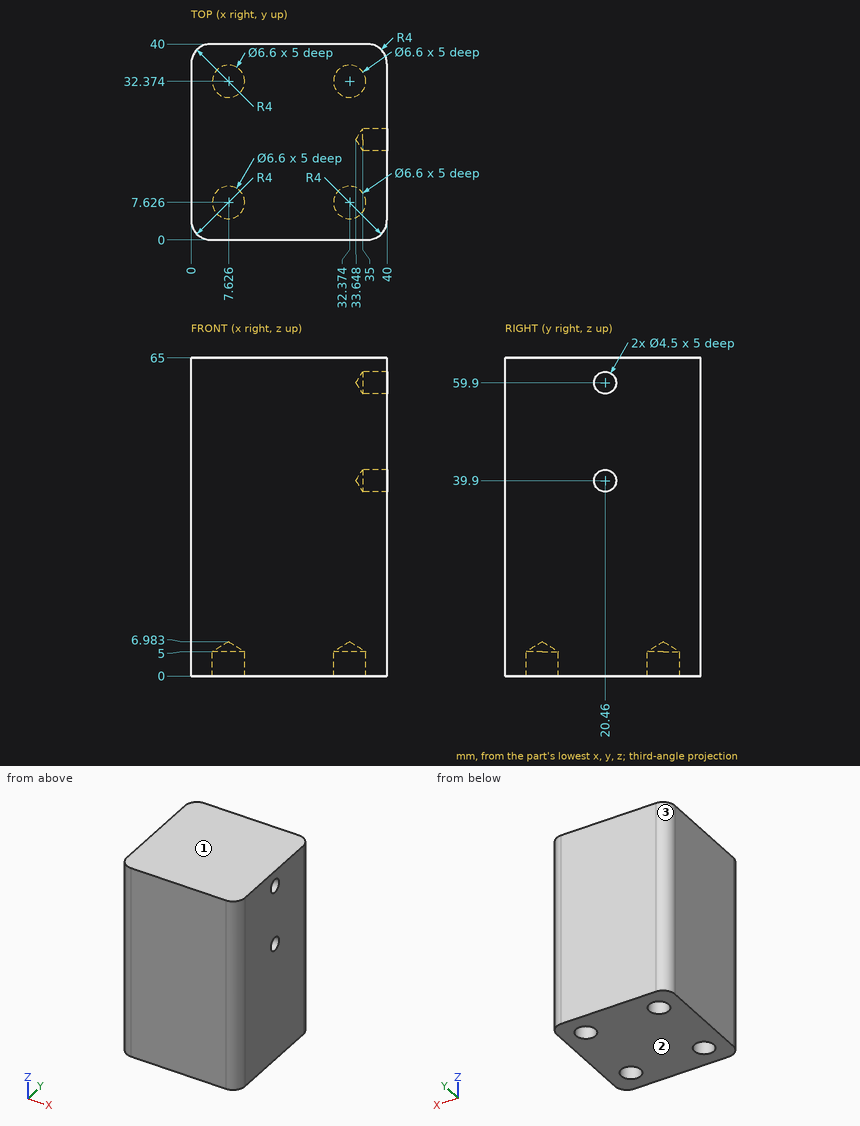
Print and shaded views of the part. All mm, measured from the part's lowest x, y and z. Coordinates: 2 decimals unless noted, no trailing zeros. Answer as a JSON object with one key per item and string values. Group by question number.
1) Flat gauge pins, fed straight in: pin 1 (5.5 mm diameter, centred on x = 7.63, y = 7.63, fed in from -Z); pin 2 (2.5 mm diameter, centred on y = 20.46, z = 39.9, fed in from +X). Where does each tip first touch, or does it go through?
2) Pull direction Z, two halves, no side cores. Call the marked faces 1, 2 and 3: +Z half, -Z half, draft (parallel to the pull), parting line (faces both ways), or undercut.
3) Drill centre lines: L1, parallel to Y at x = 38, z = 59 (1 decimal); L2, parallel to Y at x = 37, z = 59; L3, parallel to Z at x = 34, y = 7 (1 decimal). Where is each one in solid material? Low to high.
Check values:
{
 "1": {"pin 1": "stops at z = 5.33", "pin 2": "stops at x = 34.4"},
 "2": {"face 1": "+Z half", "face 2": "-Z half", "face 3": "draft"},
 "3": {"L1": "y = 0.5 to 18.4, 22.5 to 39.5", "L2": "y = 0.13 to 18.4, 22.52 to 39.87", "L3": "z = 5.9 to 65"}
}
